The model under review builds one solid part; all positions refer to its coordinate system, in mm. A direction names the side the tool comes from. Give positions to 0.01 mm unless a question says otherwise; leave off trailing zeros. Order: outer loops, then holes, each group sorted by start corner. A loop starts at its lowest first (then second) coordinate and runs counter-clockwise, first axis right, second up. Notation, with made-up numbers: (-19.5, -27.75) -> (6.5, -27.75) arc R19 cw to (6.5, -8.75) -> close; hole circle Ø11 at (26.5, -5.75). An arc over 180 degrees is marked (long way). Answer as a JSON object with one key per item and string values. Group by question number.
from build123d import *

# Parameters (mm, degrees)
SKETCH1_W           = 108
SKETCH1_H           = 38
SKETCH1_R           = 2.1
SKETCH1_W_2         = 10
SKETCH1_H_2         = 4
BOSS_EXTRUDE1_DEPTH = 4


with BuildPart() as part:
    # Sketch1 → Boss-Extrude1 (new body)
    with BuildSketch(Plane(origin=(0, 0, 0), x_dir=(1, 0, 0), z_dir=(0, 1, 0))):
        with Locations((54, 19)):
            Rectangle(SKETCH1_W, SKETCH1_H)
        with Locations(Location((5, 33, 0), (0, 0, 270))):
            Circle(SKETCH1_R, mode=Mode.SUBTRACT)
        with Locations(Location((5, 5, 0), (0, 0, 270))):
            Circle(SKETCH1_R, mode=Mode.SUBTRACT)
        with Locations(Location((103, 5, 0), (0, 0, 270))):
            Circle(SKETCH1_R, mode=Mode.SUBTRACT)
        with Locations(Location((103, 33, 0), (0, 0, 270))):
            Circle(SKETCH1_R, mode=Mode.SUBTRACT)
        with Locations((19, 12.5)):
            Rectangle(SKETCH1_W_2, SKETCH1_H_2, mode=Mode.SUBTRACT)
        with Locations((19, 25.5)):
            Rectangle(SKETCH1_W_2, SKETCH1_H_2, mode=Mode.SUBTRACT)
        with Locations((54, 25.5)):
            Rectangle(SKETCH1_W_2, SKETCH1_H_2, mode=Mode.SUBTRACT)
        with Locations((54, 12.5)):
            Rectangle(SKETCH1_W_2, SKETCH1_H_2, mode=Mode.SUBTRACT)
        with Locations((89, 25.5)):
            Rectangle(SKETCH1_W_2, SKETCH1_H_2, mode=Mode.SUBTRACT)
        with Locations((89, 12.5)):
            Rectangle(SKETCH1_W_2, SKETCH1_H_2, mode=Mode.SUBTRACT)
    extrude(amount=BOSS_EXTRUDE1_DEPTH)


solid = part.part
1. For probe 1 along Z at (x, y) = (53, 0.55); probe 2 along X at (y, z) = (3.55, -27); probe 3 along X at (y, z) = (1.95, -33), list the stretches that pass through material, from the lowest coordinate up. Write a range as [from, to].
2. Take a section at B-B on z = -33. Give the boundary of the cut face in (x, y), plus the area to 3 significant figures.
3. Machinability: for faces 4 (the flat face through (89, 2, -10.5)), 5 (the flat face through (0, 2, -19)), which of the approach directions +Z, -Z, +X, -X, +Y, -Y give a long, thin tool a straight path to every point of the face, cutting with its end or side? Answer none if there is none.
4. Draft analysis for pull direction Z (two halves, no side actions). For faces 1 (the flat face through (53, 2, -38)), 2 (the flat face through (89, 2, -27.5)), 3 (the flat face through (53, 4, -19)), state which applies: pulls with the +Z half, pulls with the -Z half, needs draft (parallel to the pull), parting line crosses it, or undercut.
5. Take a section at C-C on y = 3.4. State how many separate pieces and enclosed holes the cut face has, plus the area to 3 significant figures.
6. Take a section at A-A on x = 20.5. Give the boundary of the cut face in (y, z).
Checks:
{
 "1": {"probe 1": "z = [-38, -27.5], [-23.5, -14.5], [-10.5, 0]", "probe 2": "x = [0, 14], [24, 49], [59, 84], [94, 108]", "probe 3": "x = [0, 2.9], [7.1, 100.9], [105.1, 108]"},
 "2": {"outline": "(0, 0) -> (2.9, 0) -> (2.9, 4) -> (0, 4) -> close; (7.1, 0) -> (100.9, 0) -> (100.9, 4) -> (7.1, 4) -> close; (105.1, 0) -> (108, 0) -> (108, 4) -> (105.1, 4) -> close", "area": "398 mm2"},
 "3": {"face 4": "+Y, -Y", "face 5": "+Z, -Z, -X, +Y, -Y"},
 "4": {"face 1": "pulls with the -Z half", "face 2": "undercut", "face 3": "needs draft"},
 "5": {"separate pieces": "1", "enclosed holes": "10", "area": "3,810 mm2"},
 "6": {"outline": "(0, -38) -> (4, -38) -> (4, -27.5) -> (0, -27.5) -> close; (0, -23.5) -> (4, -23.5) -> (4, -14.5) -> (0, -14.5) -> close; (0, -10.5) -> (4, -10.5) -> (4, 0) -> (0, 0) -> close"}
}
